Autodesk Inventor part; units mm, degrees
ref_plane "YZ Plane" through (0, 0, 0) normal (1, 0, 0) x (0, 1, 0)
ref_plane "XZ Plane" through (0, 0, 0) normal (0, 1, 0) x (-1, 0, 0)
ref_plane "XY Plane" through (0, 0, 0) normal (0, 0, 1) x (1, 0, 0)
sketch "Sketch1" plane through (0, 0, 0) normal (0, 1, 0) x (-1, 0, 0)
  line L0 (8.89, 15.24) -> (-8.89, 15.24)
  line L1 (-8.89, 15.24) -> (-8.89, -15.24)
  line L2 (-8.89, -15.24) -> (8.89, -15.24)
  line L3 (8.89, -15.24) -> (8.89, 15.24)
  line L4 (8.89, 15.24) -> (-8.89, -15.24) construction
  line L5 (-8.89, 15.24) -> (8.89, -15.24) construction
  line L6 (8.89, 0) -> (8.89, -12.7)
  line L7 (8.89, 0) -> (8.89, 12.7)
  line L8 (8.89, 15.24) -> (0, 15.24)
  circle A0 centre (0, 12.7) radius 1.27
  circle A1 centre (0, -12.7) radius 1.27
  point P0 (0, 0)
  dimension "d0" = 17.78
  dimension "d1" = 30.48
  dimension "d2" = 12.7
  dimension "d3" = 12.7
  dimension "d4" = 8.89
  dimension "d5" = 2.54
  dimension "d6" = 2.54
extrude "Extrusion1" add sketch "Sketch1" along normal blind 0.762
ref_plane "Work Plane1" through (-8.89, 0, 0) normal (0, 0, 1) x (1, 0, 0)
properties part number "adafruit_TCA9548A_board" material "PET Plastic White"
Part model, mm, in its own coordinate system. Give positions to 0.01 mm unless a question says otherwise; leave off trailing zeros. Order: outer loops, then holes, each group sorted by start corner. A loop starts at its lowest first (then second) coordinate and runs counter-clockwise, first axis right, second up. Notation, with made-up numbers: M 46,5.25 L 93,5.25 A18 cw 93,10.25 Z; hole C -14.75,29 d5. An arc over 180 degrees is marked long. Use a Markdown table: item, result. Add a question column.
(1) Saw through at B-B, the plane z = 12.7. Give the cut face in (x, y).
(2) Mould opens along X. For faces 1 (the face through (0, 0, 0)), 2 (the face through (0.28, 0.38, 13.94)) say: +X half, -X half, draft (parallel to the pull), parting line (faces both ways), or undercut.
(3) Saw through at A-A, the plane x = 0. Give the cut face in (y, z).
(4) Probe line 1 along Z through (x, y) = (0, 0.3); line 2 along Z through (x, y) = (-0.25, 0.2); line 3 along X through (y, z) = (0.2, 13.5). List the from-to ranges inside material, lowest first. Write a range as [from, to].
(5) Saw through at C-C, the plane y = 0.6. Give the cut face in (x, z), and give its area (3 significant figures).
Answer key:
| question | item | result |
|---|---|---|
| 1 | outline | M -8.89,0 L -1.27,0 L -1.27,0.76 L -8.89,0.76 Z; M 1.27,0 L 8.89,0 L 8.89,0.76 L 1.27,0.76 Z |
| 2 | face 1 | draft |
| 2 | face 2 | undercut |
| 3 | outline | M 0,-15.24 L 0.76,-15.24 L 0.76,-13.97 L 0,-13.97 Z; M 0,-11.43 L 0.76,-11.43 L 0.76,11.43 L 0,11.43 Z; M 0,13.97 L 0.76,13.97 L 0.76,15.24 L 0,15.24 Z |
| 4 | line 1 | [-15.24, -13.97], [-11.43, 11.43], [13.97, 15.24] |
| 4 | line 2 | [-15.24, -13.95], [-11.45, 11.45], [13.95, 15.24] |
| 4 | line 3 | [-8.89, -0.99], [0.99, 8.89] |
| 5 | outline | M -8.89,-15.24 L 8.89,-15.24 L 8.89,15.24 L -8.89,15.24 Z; hole C 0,-12.7 d2.54; hole C 0,12.7 d2.54 |
| 5 | area | 532 mm^2 |
